Verification items for the finished model (mm, model axes). Face numbers are marked on the shaded views. A direction names the side the tool comes from. Round coordinates to 2 decimals unless told otherwise and drop trailing zeros. Loops run counter-clockwise (first coordinate to the right, second up) from the corner with the lowest first, then second, coordinate; pieces in that order, holes last. Notation, with made-up numbers: (43.25, 5) - (74.25, 5) arc R13 ccw to (74.25, 14) - close; hole circle Ø10 at (11.25, 15.5). An arc over 180 degrees is marked (long way). Use CSV: the item, a comma, the result in double quotes.
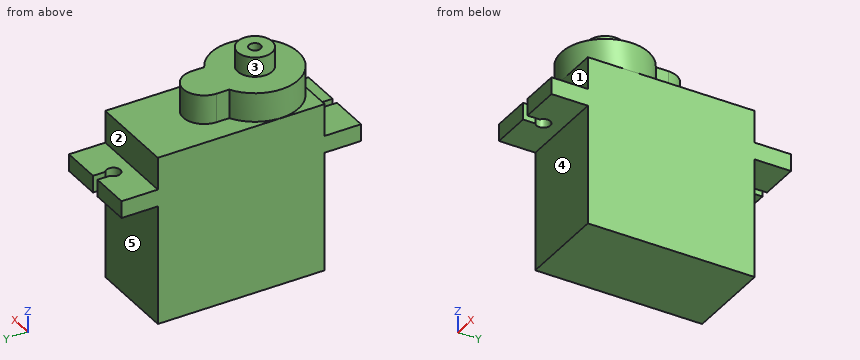
```python
from build123d import *

# Parameters (mm, degrees)
SKETCH1_W           = 12.07
SKETCH1_H           = 23.27
BOSS_EXTRUDE1_DEPTH = 23
SKETCH2_R           = 6
BOSS_EXTRUDE3_DEPTH = 4
BOSS_EXTRUDE4_DEPTH = 4
SKETCH6_W           = 12.07
SKETCH6_H           = 2.35
BOSS_EXTRUDE5_DEPTH = 5
SKETCH7_W           = 12.07
SKETCH7_H           = 2.35
BOSS_EXTRUDE6_DEPTH = 5
SKETCH8_R           = 0.95
CUT_EXTRUDE1_DEPTH  = 36.831233582
SKETCH9_W           = 1.02
SKETCH9_H           = 2.5
CUT_EXTRUDE2_DEPTH  = 36.831233582
SKETCH10_R          = 2.38
SKETCH10_R_2        = 0.815
BOSS_EXTRUDE7_DEPTH = 2.7


with BuildPart() as part:
    # Sketch1 → Boss-Extrude1 (new body)
    with BuildSketch(Plane(origin=(0, 0, 0), x_dir=(1, 0, 0), z_dir=(0, 1, 0))):
        with Locations((6.035, 11.635)):
            Rectangle(SKETCH1_W, SKETCH1_H)
    extrude(amount=BOSS_EXTRUDE1_DEPTH)

    # Sketch2 → Boss-Extrude3 (add)
    with BuildSketch(Plane.XY):
        with Locations(Location((6.035, 6, 0), (0, 0, 270))):
            Circle(SKETCH2_R)
    extrude(amount=BOSS_EXTRUDE3_DEPTH)

    # Sketch4 → Boss-Extrude4 (add)
    with BuildSketch(Plane.XY):
        with BuildLine():
            Line((3.155, 13), (3.155, 11.263610928))
            Line((3.155, 11.263610928), (8.915, 11.263610928))
            Line((8.915, 11.263610928), (8.915, 13))
            ThreePointArc((8.915, 13), (6.035, 15.88), (3.155, 13))
        make_face()
    extrude(amount=BOSS_EXTRUDE4_DEPTH)

    # Sketch6 → Boss-Extrude5 (add)
    with BuildSketch(Plane.XZ):
        with Locations((6.035, -5.625)):
            Rectangle(SKETCH6_W, SKETCH6_H)
    extrude(amount=BOSS_EXTRUDE5_DEPTH)

    # Sketch7 → Boss-Extrude6 (add)
    with BuildSketch(Plane(origin=(0, 23, 0), x_dir=(-1, 0, 0), z_dir=(0, 1, 0))):
        with Locations((-6.035, -5.625)):
            Rectangle(SKETCH7_W, SKETCH7_H)
    extrude(amount=BOSS_EXTRUDE6_DEPTH)

    # Sketch8 → Cut-Extrude1 (cut, through all)
    with BuildSketch(Plane.XY.offset(-4.45)):
        with Locations((6.035, 25.5)):
            Circle(SKETCH8_R)
        with Locations((6.035, -2.5)):
            Circle(SKETCH8_R)
    extrude(amount=-CUT_EXTRUDE1_DEPTH, mode=Mode.SUBTRACT)

    # Sketch9 → Cut-Extrude2 (cut, through all)
    with BuildSketch(Plane.XY.offset(-4.45)):
        with Locations((6.035, 26.75)):
            Rectangle(SKETCH9_W, SKETCH9_H)
        with Locations((6.035, -3.75)):
            Rectangle(SKETCH9_W, SKETCH9_H)
    extrude(amount=-CUT_EXTRUDE2_DEPTH, mode=Mode.SUBTRACT)

    # Sketch10 → Boss-Extrude7 (add)
    with BuildSketch(Plane.XY.offset(4)):
        with Locations(Location((6.035, 6, 0), (0, 0, 180))):
            Circle(SKETCH10_R)
        with Locations(Location((6.035, 6, 0), (0, 0, 180))):
            Circle(SKETCH10_R_2, mode=Mode.SUBTRACT)
    extrude(amount=BOSS_EXTRUDE7_DEPTH)


solid = part.part
```
1) Cross-section at D-D, the plane z = -8. Record the cut outline in (x, y).
Returned:
outline,"(0, 0) - (12.07, 0) - (12.07, 23) - (0, 23) - close"
2) Thickness scan on probe 1 along X at (y, z) = (6, 5.15) (3 decimals); probe 2 along X at (y, z) = (25.5, -5.8) (3 decimals); probe 3 along Z at (x, y) = (3, 17.5). Record the ranges inside material, lowest first. Write a range as [from, to].
Returned:
probe 1,"x = [3.655, 5.22], [6.85, 8.415]"
probe 2,"x = [0, 5.085], [6.985, 12.07]"
probe 3,"z = [-23.27, 0]"
3) Gauge pin test, flat ends, axial feed: pin 1 Ø1.5 at (x, y) = (4.5, 26) entering from +Z; pin 2 Ø1.7 at (x, y) = (6.035, -2.5) entering from -Z; pin 3 Ø5 at (x, z) = (3.5, -1) entering from +Y; pin 4 Ø2.5 at (x, y) = (8, -3) entering from -Z. Record the tip position at first contact, or that the pin passes through.
Returned:
pin 1,"stops at z = -4.45"
pin 2,"passes through"
pin 3,"stops at y = 23"
pin 4,"stops at z = -6.8"
4) Cross-section at A-A, the plane y = 25.5. Record the cut outline in (x, z) (3 decimals).
Returned:
outline,"(0, -6.8) - (5.085, -6.8) - (5.085, -4.45) - (0, -4.45) - close; (6.985, -6.8) - (12.07, -6.8) - (12.07, -4.45) - (6.985, -4.45) - close"
5) Access from +Z, -Z, +X, -X, +Y, -Y to the whole of each face (thin tool, end or side, straight path). Record for the marked faces 1, 2, 3, 4 and 5.
Returned:
face 1,"+Z, +X, -X, -Y"
face 2,"+Z, +X, -X, +Y"
face 3,"+Z"
face 4,"-Z, +X, -X, -Y"
face 5,"-Z, +X, -X, +Y"
6) Cross-section at C-C, the plane y = 6. Record the cut outline in (x, z) (3 decimals), then the cut area to 3 significant figures.
Returned:
outline,"(0, -23.27) - (12.07, -23.27) - (12.07, 0) - (12.035, 0) - (12.035, 4) - (8.415, 4) - (8.415, 6.7) - (6.85, 6.7) - (6.85, 4) - (5.22, 4) - (5.22, 6.7) - (3.655, 6.7) - (3.655, 4) - (0.035, 4) - (0.035, 0) - (0, 0) - close"
area,"337 mm²"
7) Cross-section at B-B, the plane x = 2.75. Record the cut outline in (y, z), then the cut area to 3 significant figures.
Returned:
outline,"(-5, -6.8) - (0, -6.8) - (0, -23.27) - (23, -23.27) - (23, -6.8) - (28, -6.8) - (28, -4.45) - (23, -4.45) - (23, 0) - (11.02, 0) - (11.02, 4) - (0.98, 4) - (0.98, 0) - (0, 0) - (0, -4.45) - (-5, -4.45) - close"
area,"599 mm²"
